```python
from build123d import *

# Parameters (mm, degrees)
SKETCH_1_W           = 160
SKETCH_1_H           = 60.5
EXTRUDE_1_DEPTH      = 5
SKETCH_2_R           = 13.45
SKETCH_2_R_2         = 1.525
CUT_EXTRUDE_1_DEPTH  = 34
SKETCH_3_R           = 2.025
CUT_EXTRUDE_2_DEPTH  = 10
SKETCH_4_R           = 1.525
CUT_EXTRUDE_3_DEPTH  = 10
SKETCH_5_W           = 160
SKETCH_5_H           = 1.5
EXTRUDE_2_DEPTH      = 5
SKETCH_6_W           = 25
SKETCH_6_H           = 24
EXTRUDE_3_DEPTH      = 5
FILLET_1_R           = 5
SKETCH_7_W           = 15
SKETCH_7_H           = 14.5
CUT_EXTRUDE_4_DEPTH  = 5
FILLET_2_R           = 2
SKETCH_8_W           = 10
SKETCH_8_H           = 12
EXTRUDE_4_DEPTH      = 5
CUT_EXTRUDE_5_DEPTH  = 5
SKETCH_12_R          = 2.025
CUT_EXTRUDE_6_DEPTH  = 10
CUT_EXTRUDE_7_DEPTH  = 10
CUT_EXTRUDE_8_DEPTH  = 10
FILLET_3_R           = 2
FILLET_4_R           = 2
SKETCH_15_R          = 1.525
CUT_EXTRUDE_9_DEPTH  = 10
SKETCH_16_R          = 2.025
CUT_EXTRUDE_10_DEPTH = 10
SKETCH_17_R          = 1.525
CUT_EXTRUDE_11_DEPTH = 10
SKETCH_19_R          = 2.025
CUT_EXTRUDE_12_DEPTH = 10


with BuildPart() as part:
    # 草图1 → 凸台-拉伸1 (new body)
    with BuildSketch(Plane.XY):
        Rectangle(SKETCH_1_W, SKETCH_1_H)
    extrude(amount=EXTRUDE_1_DEPTH)

    # 草图2 → 切除-拉伸1 (cut)
    with BuildSketch(Plane.XY.offset(5)):
        with Locations((36.5, 1.25)):
            Circle(SKETCH_2_R)
        with Locations((36.5, 18.75)):
            Circle(SKETCH_2_R_2)
        with Locations((45.25, 16.405444566)):
            Circle(SKETCH_2_R_2)
        with Locations((51.655444566, 10)):
            Circle(SKETCH_2_R_2)
        with Locations((54, 1.25)):
            Circle(SKETCH_2_R_2)
        with Locations((51.655444566, -7.5)):
            Circle(SKETCH_2_R_2)
        with Locations((45.25, -13.905444566)):
            Circle(SKETCH_2_R_2)
        with Locations((36.5, -16.25)):
            Circle(SKETCH_2_R_2)
        with Locations((27.75, -13.905444566)):
            Circle(SKETCH_2_R_2)
        with Locations((21.344555434, -7.5)):
            Circle(SKETCH_2_R_2)
        with Locations((19, 1.25)):
            Circle(SKETCH_2_R_2)
        with Locations((21.344555434, 10)):
            Circle(SKETCH_2_R_2)
        with Locations((27.75, 16.405444566)):
            Circle(SKETCH_2_R_2)
    cut_extrude_1 = extrude(amount=-CUT_EXTRUDE_1_DEPTH, mode=Mode.SUBTRACT)

    # 镜向1: 切除-拉伸1 across plane
    add(cut_extrude_1.mirror(Plane(origin=(0, 0, 0), x_dir=(0, 0, 1), z_dir=(1, 0, 0))), mode=Mode.SUBTRACT)

    # 草图3 → 切除-拉伸2 (cut)
    with BuildSketch(Plane.XY.offset(5)):
        with Locations((-12, 26.25)):
            Circle(SKETCH_3_R)
        with Locations((0, 1.25)):
            Circle(SKETCH_3_R)
        with Locations((12, 26.25)):
            Circle(SKETCH_3_R)
    extrude(amount=-CUT_EXTRUDE_2_DEPTH, mode=Mode.SUBTRACT)

    # 草图4 → 切除-拉伸3 (cut)
    with BuildSketch(Plane.XY.offset(5)):
        with Locations((7.5, -27.25)):
            Circle(SKETCH_4_R)
        with Locations((-7.5, -27.25)):
            Circle(SKETCH_4_R)
    extrude(amount=-CUT_EXTRUDE_3_DEPTH, mode=Mode.SUBTRACT)

    # 草图5 → 凸台-拉伸2 (add)
    with BuildSketch(Plane.XY.offset(5)):
        with Locations((0, -31)):
            Rectangle(SKETCH_5_W, SKETCH_5_H)
    extrude(amount=-EXTRUDE_2_DEPTH)

    # 草图6 → 凸台-拉伸3 (add)
    with BuildSketch(Plane.XY.offset(5)):
        with Locations((51.5, -31.75)):
            Rectangle(SKETCH_6_W, SKETCH_6_H)
    extrude_3 = extrude(amount=-EXTRUDE_3_DEPTH)

    # 镜向2: 凸台-拉伸3 across plane
    add(extrude_3.mirror(Plane(origin=(0, 0, 0), x_dir=(0, 0, 1), z_dir=(1, 0, 0))))

    # 圆角1
    fillet_1_edges = [part.edges().sort_by_distance(p)[0] for p in [
        (64, -31.75, 2.5),
        (39, -31.75, 2.5),
        (39, -43.75, 2.5),
        (64, -43.75, 2.5),
        (-64, -31.75, 2.5),
        (-39, -31.75, 2.5),
        (-64, -43.75, 2.5),
        (-39, -43.75, 2.5),
    ]]
    fillet(fillet_1_edges, radius=FILLET_1_R)

    # 草图7 → 切除-拉伸4 (cut)
    with BuildSketch(Plane.XY.offset(5)):
        with Locations((51.5, -31.5)):
            Rectangle(SKETCH_7_W, SKETCH_7_H)
    cut_extrude_4 = extrude(amount=-CUT_EXTRUDE_4_DEPTH, mode=Mode.SUBTRACT)

    # 镜向3: 切除-拉伸4 across plane
    add(cut_extrude_4.mirror(Plane(origin=(0, 0, 0), x_dir=(0, 0, 1), z_dir=(1, 0, 0))), mode=Mode.SUBTRACT)

    # 圆角2
    fillet_2_edges = [part.edges().sort_by_distance(p)[0] for p in [
        (44, -24.25, 2.5),
        (44, -38.75, 2.5),
        (59, -38.75, 2.5),
        (59, -24.25, 2.5),
        (-59, -38.75, 2.5),
        (-59, -24.25, 2.5),
        (-44, -24.25, 2.5),
        (-44, -38.75, 2.5),
    ]]
    fillet(fillet_2_edges, radius=FILLET_2_R)

    # 草图8 → 凸台-拉伸4 (add)
    with BuildSketch(Plane(origin=(0, 0, 0), x_dir=(-1, 0, 0), z_dir=(0, 0, -1))):
        with Locations((-60.2, 36.25)):
            Rectangle(SKETCH_8_W, SKETCH_8_H)
    extrude_4 = extrude(amount=-EXTRUDE_4_DEPTH)

    # 镜向4: 凸台-拉伸4 across plane
    add(extrude_4.mirror(Plane(origin=(0, 0, 0), x_dir=(0, 0, 1), z_dir=(1, 0, 0))))

    # 草图11 → 切除-拉伸5 (cut)
    with BuildSketch(Plane(origin=(0, 0, 0), x_dir=(-1, 0, 0), z_dir=(0, 0, -1))):
        Polygon((-65.2, 30.25), (-80, 8.25), (-80, 30.25), align=None)
        Polygon((80, 30.25), (65.2, 30.25), (80, 8.25), align=None)
    extrude(amount=-CUT_EXTRUDE_5_DEPTH, mode=Mode.SUBTRACT)

    # 草图12 → 切除-拉伸6 (cut)
    with BuildSketch(Plane(origin=(0, 0, 0), x_dir=(-1, 0, 0), z_dir=(0, 0, -1))):
        with Locations((75, 4.25)):
            Circle(SKETCH_12_R)
        with Locations((75, -27.75)):
            Circle(SKETCH_12_R)
        with Locations((-75, -27.75)):
            Circle(SKETCH_12_R)
        with Locations((-75, 4.25)):
            Circle(SKETCH_12_R)
    extrude(amount=-CUT_EXTRUDE_6_DEPTH, mode=Mode.SUBTRACT)

    # 草图13 → 切除-拉伸7 (cut)
    with BuildSketch(Plane(origin=(0, 0, 0), x_dir=(-1, 0, 0), z_dir=(0, 0, -1))):
        with BuildLine():
            Line((-10.269060233, 22.25), (-18.720728361, 13.25))
            ThreePointArc((-18.720728361, 13.25), (-16.665960567, 9.417825889), (-15.426260417, 5.25))
            Line((-15.426260417, 5.25), (15.426260417, 5.25))
            ThreePointArc((15.426260417, 5.25), (16.665960567, 9.417825889), (18.720728361, 13.25))
            Line((18.720728361, 13.25), (10.269060233, 22.25))
            Line((10.269060233, 22.25), (-10.269060233, 22.25))
        make_face()
    extrude(amount=-CUT_EXTRUDE_7_DEPTH, mode=Mode.SUBTRACT)

    # 草图14 → 切除-拉伸8 (cut)
    with BuildSketch(Plane(origin=(0, 0, 0), x_dir=(-1, 0, 0), z_dir=(0, 0, -1))):
        with BuildLine():
            Line((-15.426260417, -2.75), (15.426260417, -2.75))
            ThreePointArc((15.426260417, -2.75), (17.096450252, -7.893563703), (20, -12.455929374))
            Line((20, -12.455929374), (20, -24.25))
            Line((20, -24.25), (-20, -24.25))
            Line((-20, -24.25), (-20, -12.455929374))
            ThreePointArc((-20, -12.455929374), (-17.096450252, -7.893563703), (-15.426260417, -2.75))
        make_face()
    extrude(amount=-CUT_EXTRUDE_8_DEPTH, mode=Mode.SUBTRACT)

    # 圆角3
    fillet_3_edges = [part.edges().sort_by_distance(p)[0] for p in [
        (10.269060233, 22.25, 2.5),
        (-10.269060233, 22.25, 2.5),
        (-18.720728361, 13.25, 2.5),
        (-15.426260417, 5.25, 2.5),
        (15.426260417, 5.25, 2.5),
        (18.720728361, 13.25, 2.5),
        (20, -12.455929374, 2.5),
        (15.426260417, -2.75, 2.5),
        (-15.426260417, -2.75, 2.5),
        (-20, -12.455929374, 2.5),
        (-20, -24.25, 2.5),
        (20, -24.25, 2.5),
    ]]
    fillet(fillet_3_edges, radius=FILLET_3_R)

    # 圆角4
    fillet_4_edges = [part.edges().sort_by_distance(p)[0] for p in [
        (80, -31.75, 2.5),
        (-80, -31.75, 2.5),
        (65.2, 42.25, 2.5),
        (55.2, 42.25, 2.5),
        (55.2, 30.25, 2.5),
        (65.2, 30.25, 2.5),
        (-55.2, 30.25, 2.5),
        (-65.2, 30.25, 2.5),
        (-65.2, 42.25, 2.5),
        (-55.2, 42.25, 2.5),
        (80, 8.25, 2.5),
        (-80, 8.25, 2.5),
    ]]
    fillet(fillet_4_edges, radius=FILLET_4_R)

    # 草图15 → 切除-拉伸9 (cut)
    with BuildSketch(Plane.XY.offset(5)):
        with Locations((-65, 1.750036)):
            Circle(SKETCH_15_R)
        with Locations((-65, -18.249964)):
            Circle(SKETCH_15_R)
        with Locations(Location((65, -18.249964, 0), (0, 0, 180))):
            Circle(SKETCH_15_R)
        with Locations(Location((65, 1.750036, 0), (0, 0, 180))):
            Circle(SKETCH_15_R)
    extrude(amount=-CUT_EXTRUDE_9_DEPTH, mode=Mode.SUBTRACT)

    # 草图16 → 切除-拉伸10 (cut)
    with BuildSketch(Plane(origin=(0, 0, 0), x_dir=(-1, 0, 0), z_dir=(0, 0, -1))):
        with Locations((-59.2, 37.25)):
            Circle(SKETCH_16_R)
    cut_extrude_10 = extrude(amount=-CUT_EXTRUDE_10_DEPTH, mode=Mode.SUBTRACT)

    # 镜向5: 切除-拉伸10 across plane
    add(cut_extrude_10.mirror(Plane(origin=(0, 0, 0), x_dir=(0, 0, 1), z_dir=(1, 0, 0))), mode=Mode.SUBTRACT)

    # 草图17 → 切除-拉伸11 (cut)
    with BuildSketch(Plane(origin=(0, 0, 0), x_dir=(-1, 0, 0), z_dir=(0, 0, -1))):
        with Locations((-59.2, 22.25)):
            Circle(SKETCH_17_R)
        with Locations((-67.572650385, 9.804168347)):
            Circle(SKETCH_17_R)
    cut_extrude_11 = extrude(amount=-CUT_EXTRUDE_11_DEPTH, mode=Mode.SUBTRACT)

    # 镜向6: 切除-拉伸11 across plane
    add(cut_extrude_11.mirror(Plane(origin=(0, 0, 0), x_dir=(0, 0, 1), z_dir=(1, 0, 0))), mode=Mode.SUBTRACT)

    # 草图19 → 切除-拉伸12 (cut)
    with BuildSketch(Plane(origin=(0, 0, 0), x_dir=(-1, 0, 0), z_dir=(0, 0, -1))):
        with Locations((-75, -5.75)):
            Circle(SKETCH_19_R)
        with Locations((-75, -17.75)):
            Circle(SKETCH_19_R)
        with Locations((75, -17.75)):
            Circle(SKETCH_19_R)
        with Locations((75, -5.75)):
            Circle(SKETCH_19_R)
    extrude(amount=-CUT_EXTRUDE_12_DEPTH, mode=Mode.SUBTRACT)


solid = part.part
```
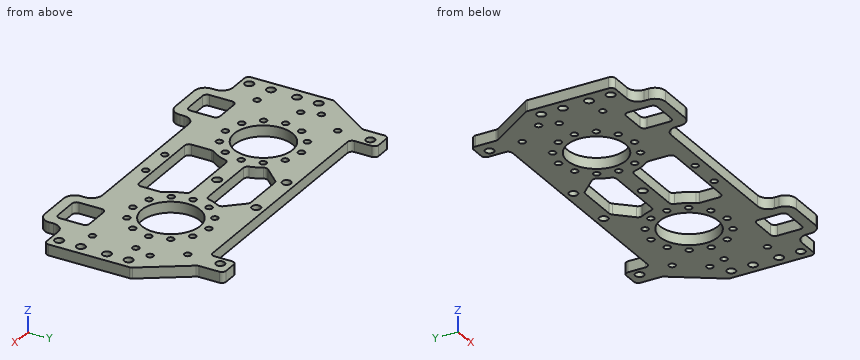
Build history of the part. All positions in model axes, mm. Round coordinates to 2 decimals unless told otherwise and drop trailing zeros. Write each loop counter-clockwise with the first axis right and the second up, starting at its lowest first coordinate (ties: lowest second). Pieces come first, ordered by that corner, then holes. Notation, with made-up numbers: (31.25, 44.25) -> (37.25, 44.25) arc R13 ccw to (37.25, 62.25) -> close; hole circle Ø7 at (19.25, 25). An arc over 180 degrees is marked (long way). Put each result on its own line as item: value.
Item 1: Wall check: probe 1 along X at (y, z) = (37, 2.3); probe 2 along Y at (x, z) = (75, 1.3) (3 decimals); probe 3 along Y at (x, z) = (55, 1.6). Give the ranges that are in metal, low to high. Write a range as from..to.
Here are the results:
probe 1: x = -65.2..-61.21, -57.19..-55.2, 55.2..57.19, 61.21..65.2
probe 2: y = -31.75..-29.775, -25.725..-19.775, -15.725..-7.775, -3.725..2.225, 6.275..15.682
probe 3: y = -43.75..-38.75, -24.25..0.1, 2.4..31.38
Item 2: Slice it at B-B, the plane z = 1.2. Count the separate pieces of the cut face and the enclosed holes in it, plus the area to 3 significant figures.
Here are the results:
separate pieces: 1
enclosed holes: 53
area: 7,120 mm^2
Item 3: Flat gauge pins, fed straight in: P1, Ø2.5, axis at x = -75, y = -27.75, coming from the +Z side; P2, Ø2, axis at y = -37.5, z = 3.5, coming from the +X side; P3, Ø2, axis at x = 40, z = 3, coming from the +Y side. Where does each tip first touch, or does it go through?
Here are the results:
P1: passes through
P2: stops at x = 64.01
P3: stops at y = 30.25
Item 4: Slice it at A-A, the plane x = 0. Give the cut face in (y, z) (3 decimals), plus the area to 4 significant figures.
Here are the results:
outline: (-31.75, 0) -> (-24.25, 0) -> (-24.25, 5) -> (-31.75, 5) -> close; (-2.75, 0) -> (-0.775, 0) -> (-0.775, 5) -> (-2.75, 5) -> close; (3.275, 0) -> (5.25, 0) -> (5.25, 5) -> (3.275, 5) -> close; (22.25, 0) -> (30.25, 0) -> (30.25, 5) -> (22.25, 5) -> close
area: 97.25 mm^2
